```python
from build123d import *

# Parameters (mm, degrees)
F0_W     = 450.85
F0_H     = 355.6
F1_DEPTH = 19.05
F3_D     = 38.1
F5_D     = 9.525
F6_W     = 15.875
F6_H     = 57.15
F7_DEPTH = 139.7


# Not quite as in the source:
# - a length typed as a fraction of an inch, garbled in the dataset ("3 / 203.2 mm" for 3/8 in), is restored


with BuildPart() as f1:
    # F0 (on Top) → F1 (new body)
    with BuildSketch(Plane.XY):
        Rectangle(F0_W, F0_H)
    extrude(amount=F1_DEPTH)

    # F3 (through all)
    with Locations(Plane.XY.offset(19.05)):
        with Locations((25.4, 76.2), (25.4, -88.9)):
            Hole(F3_D / 2)

    # F5 (through all)
    with Locations(Plane(origin=(0, 0, 0), x_dir=(1, 0, 0), z_dir=(0, 0, -1))):
        with Locations((0, 160.3375), (0, -160.3375)):
            Hole(F5_D / 2)

    # F6 (on Front) → F7 (join, symmetric)
    with BuildSketch(Plane.XZ):
        with Locations((207.9625, -28.575)):
            Rectangle(F6_W, F6_H)
        with Locations((-1.5875, -28.575)):
            Rectangle(F6_W, F6_H)
        with Locations((-207.9625, -28.575)):
            Rectangle(F6_W, F6_H)
    extrude(amount=F7_DEPTH, both=True)


solid = f1.part
```
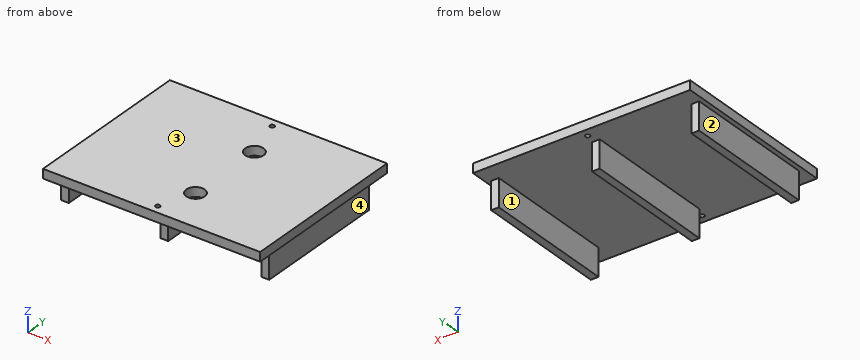
Check sheet for the modelled part. Datum: model origin and axes. Units: mm. Face numbers are marked on the shaded views. A direction names the side the tool comes from. Round coordinates to 2 decimals unless told otherwise and drop trailing zeros. Loops run counter-clockwise (first coordinate to the right, second up) from the corner with the lowest first, then second, coordinate; pieces in that order, holes last. Notation, with made-up numbers: (-30, 50.25) -> (13, 50.25) arc R12 ccw to (13, 69.25) -> close; hole circle Ø8 at (-33, -24). An arc over 180 degrees is marked (long way). Answer in a Markdown table with one row per item.
Q1. Sectioned sample at D-D on y = -97. Enter the section's corners in (x, z) (3 decimals).
Data:
| item | result |
|---|---|
| outline | (-225.425, 0) -> (-215.9, 0) -> (-215.9, -57.15) -> (-200.025, -57.15) -> (-200.025, 0) -> (-9.525, 0) -> (-9.525, -57.15) -> (6.35, -57.15) -> (6.35, 0) -> (8.158, 0) -> (8.158, 19.05) -> (-225.425, 19.05) -> close; (42.642, 0) -> (200.025, 0) -> (200.025, -57.15) -> (215.9, -57.15) -> (215.9, 0) -> (225.425, 0) -> (225.425, 19.05) -> (42.642, 19.05) -> close |
Q2. Sectioned sample at B-B on x = 0. Enter the section's corners in (y, z) (3 decimals), then the cut area to 3 significant figures.
Data:
| item | result |
|---|---|
| outline | (-177.8, 0) -> (-165.1, 0) -> (-165.1, 19.05) -> (-177.8, 19.05) -> close; (-155.575, 0) -> (-139.7, 0) -> (-139.7, -57.15) -> (139.7, -57.15) -> (139.7, 0) -> (155.575, 0) -> (155.575, 19.05) -> (-155.575, 19.05) -> close; (165.1, 0) -> (177.8, 0) -> (177.8, 19.05) -> (165.1, 19.05) -> close |
| area | 22,400 mm^2 |
Q3. Sectioned sample at C-C on y = -6. Enter the section's corners in (x, z) (3 decimals), then the cut area to 3 significant figures.
Data:
| item | result |
|---|---|
| outline | (-225.425, 0) -> (-215.9, 0) -> (-215.9, -57.15) -> (-200.025, -57.15) -> (-200.025, 0) -> (-9.525, 0) -> (-9.525, -57.15) -> (6.35, -57.15) -> (6.35, 0) -> (200.025, 0) -> (200.025, -57.15) -> (215.9, -57.15) -> (215.9, 0) -> (225.425, 0) -> (225.425, 19.05) -> (-225.425, 19.05) -> close |
| area | 11,300 mm^2 |
Q4. Sectioned sample at A-A on z = -47.5. Enter the section's corners in (x, y) (3 decimals).
Data:
| item | result |
|---|---|
| outline | (-215.9, -139.7) -> (-200.025, -139.7) -> (-200.025, 139.7) -> (-215.9, 139.7) -> close; (-9.525, -139.7) -> (6.35, -139.7) -> (6.35, 139.7) -> (-9.525, 139.7) -> close; (200.025, -139.7) -> (215.9, -139.7) -> (215.9, 139.7) -> (200.025, 139.7) -> close |
Q5. Thickness scan on L1, parallel to X at y = 98.5, z = -18 (3 decimals); L2, parallel to Y at x = 25, z = 13. Record the ranges inside material, lowest first.
Data:
| item | result |
|---|---|
| L1 | x = -215.9 to -200.025, -9.525 to 6.35, 200.025 to 215.9 |
| L2 | y = -177.8 to -107.95, -69.85 to 57.15, 95.25 to 177.8 |
Q6. Set-up check for the marked faces 1, 2, 3 and 4: record each of +Z, -Z, +X, -X, +Y, -Y from which the full face is reachable in a straight line by a thin tool's end or side.
Data:
| item | result |
|---|---|
| face 1 | -Z, +Y, -Y |
| face 2 | -Z, -X, +Y, -Y |
| face 3 | +Z, +X, -X, +Y, -Y |
| face 4 | -Z, +X, +Y, -Y |
Q7. Go/stop test with flat-tipped pins: P1, Ø4, axis at y = -80.5, z = -3.5, coming from the +X side; P2, Ø12.5, axis at x = -211, z = -21, coming from the +Y side; P3, Ø15, axis at x = 0, y = -160.34, coming from the -Z side; P4, Ø15, axis at x = 0, y = 160.34, coming from the +Z side. Record where each tip stops, or that it passes through.
Data:
| item | result |
|---|---|
| P1 | stops at x = 215.9 |
| P2 | stops at y = 139.7 |
| P3 | stops at z = 0 |
| P4 | stops at z = 19.05 |
